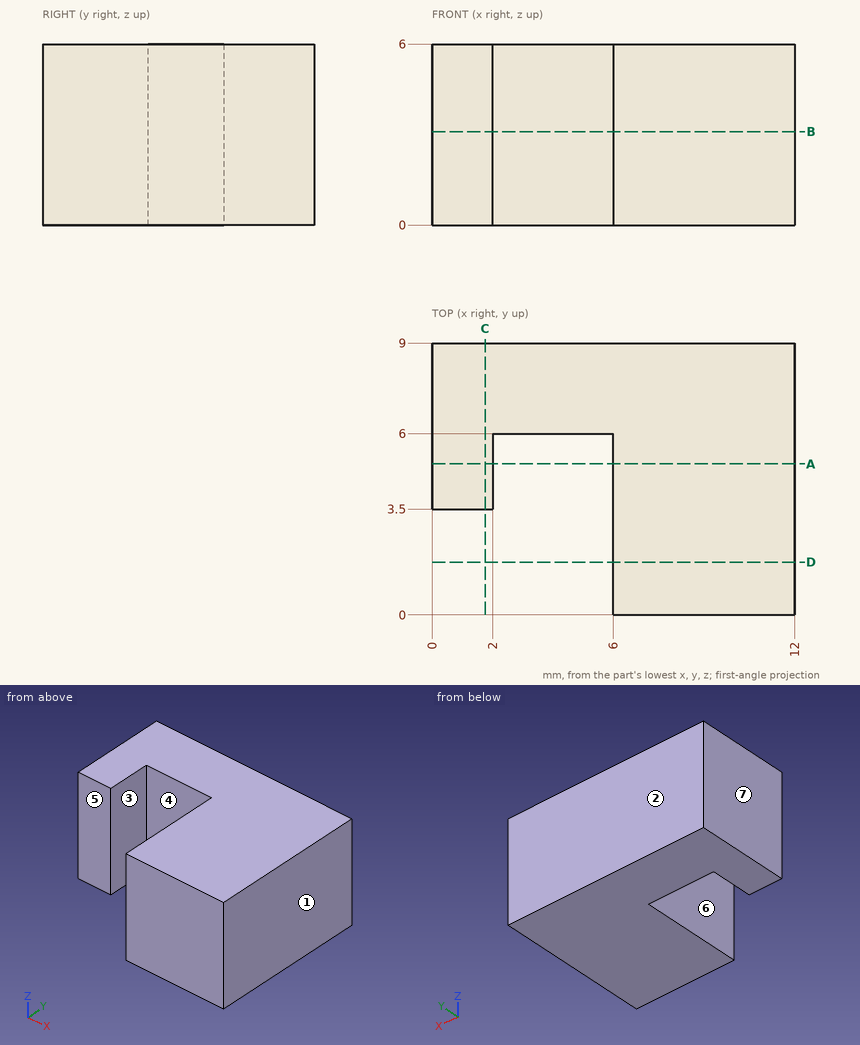
The figure shows three views and two pictorial views of one solid part (mm, origin at its lowest corner). Answer the questions. A direction names the side the tool comes from. Give positions to 0.01 mm unless a question says otherwise; leave off trailing zeros. Loops run counter-clockwise (first coordinate to the right, second up) from the corner with the lowest first, then second, coordinate; pieces in that order, holes last. Notation, with made-up numbers: (47, 79.5) -> (100, 79.5) arc R26 cw to (100, 106.5) -> close; hole circle Ø1 at (-33, -23.75). An arc over 180 degrees is marked (long way). Use a Markdown table: item, result. Add a question column.
1. Find the intervals of material crossed by probe 1 along X at (y, z) = (4, 3.7); probe 2 along X at (y, z) = (0.75, 5.6); probe 3 along Y at (x, z) = (5.5, 0.5), in increasing order.
2. For the marked faces 5, 6 and 7, determine the directions among +Z, -Z, +X, -X, +Y, -Y from which every point of the face is accessible in a straight line to the end or side of a thin tool.
3. Section D-D on y = 1.75 is taken. Determine the outline of the cut face in (x, z).
4. Determine the mould class of the marked faces 1, 2, 3 and 4 for opening direction X: released by +X, released by -X, zero draft, split by the parting line, or undercut.
5. Section B-B on z = 3.1 is taken. Determine the outline of the cut face in (x, y).
6. Section A-A on y = 5 is taken. Determine the outline of the cut face in (x, z), and give its area (3 significant figures).
7. Section C-C on x = 1.75 is taken. Determine the outline of the cut face in (y, z).
8. Flat-ended cylindrical pins translate along their axes: pin 1 Ø1.6 at (x, z) = (1.5, 4) entering from -Y; pin 2 Ø1.5 at (x, y) = (4.5, 3.5) entering from -Z. Find the tip coordinate at first contact, or state that the pin passes through.
Results below:
| question | item | result |
|---|---|---|
| 1 | probe 1 | x = 0 to 2, 6 to 12 |
| 1 | probe 2 | x = 6 to 12 |
| 1 | probe 3 | y = 6 to 9 |
| 2 | face 5 | +Z, -Z, -X, -Y |
| 2 | face 6 | +Z, -Z, -Y |
| 2 | face 7 | +Z, -Z, -X, +Y, -Y |
| 3 | outline | (6, 0) -> (12, 0) -> (12, 6) -> (6, 6) -> close |
| 4 | face 1 | released by +X |
| 4 | face 2 | zero draft |
| 4 | face 3 | undercut |
| 4 | face 4 | undercut |
| 5 | outline | (0, 3.5) -> (2, 3.5) -> (2, 6) -> (6, 6) -> (6, 0) -> (12, 0) -> (12, 9) -> (0, 9) -> close |
| 6 | outline | (0, 0) -> (2, 0) -> (2, 6) -> (0, 6) -> close; (6, 0) -> (12, 0) -> (12, 6) -> (6, 6) -> close |
| 6 | area | 48.0 mm^2 |
| 7 | outline | (3.5, 0) -> (9, 0) -> (9, 6) -> (3.5, 6) -> close |
| 8 | pin 1 | stops at y = 3.5 |
| 8 | pin 2 | passes through |
